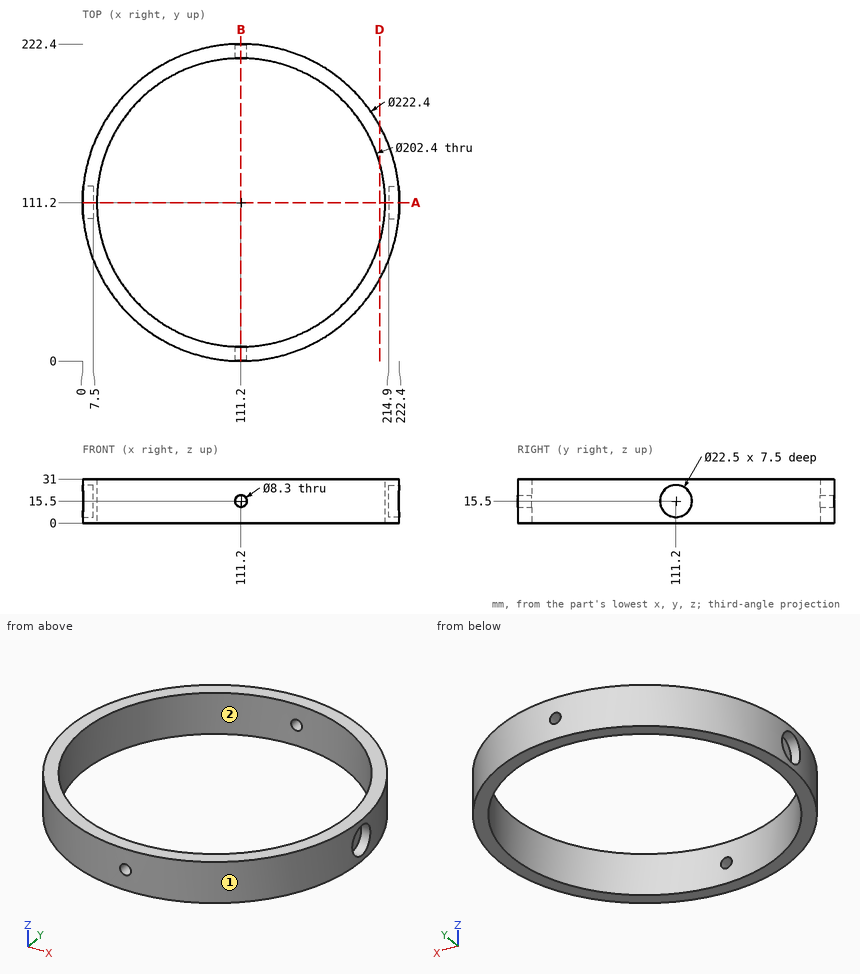
The figure shows three views and two pictorial views of one solid part (mm, origin at its lowest corner). Answer the questions. Round coordinates to 2 decimals unless told otherwise and drop trailing zeros. Order: outer loops, then holes, each group sorted by start corner. A loop starts at its lowest first (then second) coordinate and runs counter-clockwise, first axis right, second up. Notation, with made-up numbers: (21, -12.5) -> (26, -12.5) arc R18 ccw to (26, -6.5) -> close; hole circle Ø1 at (-12.5, 67.25). An arc over 180 degrees is marked (long way). Put each result on its own line as item: value.
Q1. Section B-B, the plane x = 111.2 is taken. Write down the section's boundary in (y, z), and give its area (3 significant figures).
Results list:
outline: (0, 0) -> (10, 0) -> (10, 11.35) -> (0, 11.35) -> close; (0, 19.65) -> (10, 19.65) -> (10, 31) -> (0, 31) -> close; (212.4, 0) -> (222.4, 0) -> (222.4, 11.35) -> (212.4, 11.35) -> close; (212.4, 19.65) -> (222.4, 19.65) -> (222.4, 31) -> (212.4, 31) -> close
area: 454 mm^2
Q2. Each of these flat-tipped pins is pushed along its axis until it touches: P1, Ø1.5, axis at y = 73, z = 6, coming from the +X side; P2, Ø18, axis at y = 108.5, z = 14, coming from the +X side; P3, Ø18, axis at y = 111.2, z = 15.5, coming from the +X side; P4, Ø5, axis at x = 111.2, z = 15.5, coming from the +Y side. Where does it stop, or does it pass through?
Results list:
P1: x = 215.9
P2: x = 222.31
P3: x = 214.9
P4: through
Q3. Section A-A, the plane y = 111.2 is taken. Write down the section's boundary in (x, z).
Results list:
outline: (0, 0) -> (10, 0) -> (10, 31) -> (0, 31) -> (0, 26.75) -> (7.5, 26.75) -> (7.5, 4.25) -> (0, 4.25) -> close; (212.4, 0) -> (222.4, 0) -> (222.4, 4.25) -> (214.9, 4.25) -> (214.9, 26.75) -> (222.4, 26.75) -> (222.4, 31) -> (212.4, 31) -> close
Q4. Section D-D, the plane x = 208.5 is taken. Write down the section's boundary in (y, z).
Results list:
outline: (57.37, 0) -> (83.38, 0) -> (83.38, 31) -> (57.37, 31) -> close; (139.02, 0) -> (165.03, 0) -> (165.03, 31) -> (139.02, 31) -> close
Q5. Consider line 1 along Z through (x, y) = (111.2, 215.75); line 2 along X through (y, z) = (112.5, 2); line 3 along X through (y, z) = (111, 22). Determine where each line is inside the solid, lowest interval first.
Results list:
line 1: 0 to 11.35, 19.65 to 31
line 2: 0.01 to 10.01, 212.39 to 222.39
line 3: 7.5 to 10, 212.4 to 214.9
Q6. Determine the mould class of the marked faces 1 and 2 for opening direction X: pulls with the +X half, pulls with the -X half, needs draft (parallel to the pull), parting line crosses it, or undercut.
Results list:
face 1: parting line crosses it
face 2: undercut
